Part print with two shaded views. Sizes in mm from the minimum x, y, z corner. A direction names the side the tool comes from. Round coordinates to 2 decimals unless told otherwise and drop trailing zeros. Loops run counter-clockwise (first coordinate to the right, second up) from the corner with the lowest first, then second, coordinate; pieces in that order, holes last. Notation, with made-up numbers: (64, -9.75) -> (80, -9.75) arc R21 cw to (80, -4.75) -> close; hole circle Ø7 at (-37.75, 38). An arc over 180 degrees is marked (long way). Use a Markdown table: item, result. Add a question column.
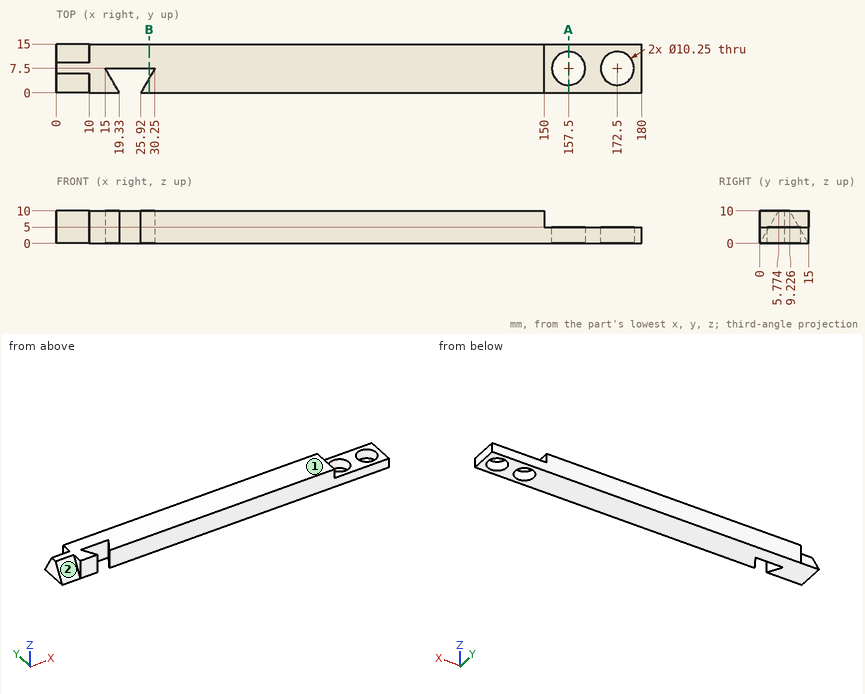
1) Pin check, flat tips, straight feed: pin 1 Ø7.5 at (x, y) = (168, 9) entering from +Z; pin 2 Ø1.7 at (y, z) = (13, 6) entering from -X. Stop position of each tip, or through.
2) Wall check: probe 1 along X at (y, z) = (8, 4.5); probe 2 along Y at (x, z) = (157.5, 1.6) (1 decimal); probe 3 along X at (y, z) = (11.25, 8.25). Give the ranges that are in metal, low to high. Write a range as from..to.
3) Cut at B-B on x = 28.5. Write the cut outline in (y, z), and give its area (3 significant figures).
4) Cut at A-A on x = 157.5. Write the cut outline in (y, z) (1 decimal).
5) Tool access for the marked faces 1 and 2: list every direction of +Z, -Z, +X, -X, +Y, -Y with a clear straight run to the whole face (end or side of a thin tool).
Established:
| question | item | result |
|---|---|---|
| 1 | pin 1 | stops at z = 5 |
| 1 | pin 2 | stops at x = 10 |
| 2 | probe 1 | x = 0..152.4, 162.6..167.4, 177.6..180 |
| 2 | probe 2 | y = 0..2.4, 12.6..15 |
| 2 | probe 3 | x = 10..150 |
| 3 | outline | (0, 0) -> (4.47, 0) -> (4.47, 10) -> (0, 10) -> close; (7.5, 0) -> (15, 0) -> (15, 10) -> (7.5, 10) -> close |
| 3 | area | 120 mm^2 |
| 4 | outline | (0, 0) -> (2.4, 0) -> (2.4, 5) -> (0, 5) -> close; (12.6, 0) -> (15, 0) -> (15, 5) -> (12.6, 5) -> close |
| 5 | face 1 | +Z, +X, -X, +Y, -Y |
| 5 | face 2 | +Z, -X, -Y |
